```python
from build123d import *
from OCP.BRepFilletAPI import BRepFilletAPI_MakeChamfer

# Parameters (mm, degrees)
SKICA1_W                = 84
SKICA1_H                = 84
P_IDAT_VYSUNUT_M1_DEPTH = 2
SKICA1_3_W              = 80
SKICA1_3_H              = 80
SKICA1_3_W_2            = 37.6
SKICA1_3_H_2            = 76.8
SKICA1_3_H_3            = 37.6
P_IDAT_VYSUNUT_M2_DEPTH = 10.8
SKICA1_4_W              = 84
SKICA1_4_H              = 84
SKICA1_4_W_2            = 80
SKICA1_4_H_2            = 80
P_IDAT_VYSUNUT_M3_DEPTH = 4
ZKOSEN_2_SIZE           = 3.464101615
ZKOSEN_2_SIZE_2         = 2


with BuildPart() as part:
    # Skica1 → Přidat vysunutím1 (new body)
    with BuildSketch(Plane(origin=(0, 0, 0), x_dir=(1, 0, 0), z_dir=(0, 1, 0))):
        with Locations((-42, 42)):
            Rectangle(SKICA1_W, SKICA1_H)
    extrude(amount=P_IDAT_VYSUNUT_M1_DEPTH)

    # Skica1<3> → Přidat vysunutím2 (add)
    with BuildSketch(Plane(origin=(0, 0, 0), x_dir=(1, 0, 0), z_dir=(0, 1, 0))):
        with Locations((-42, 42)):
            Rectangle(SKICA1_3_W, SKICA1_3_H)
        with Locations((-22.4, 42)):
            Rectangle(SKICA1_3_W_2, SKICA1_3_H_2, mode=Mode.SUBTRACT)
        with Locations((-61.6, 61.6)):
            Rectangle(SKICA1_3_W_2, SKICA1_3_H_3, mode=Mode.SUBTRACT)
        with Locations((-61.6, 22.4)):
            Rectangle(SKICA1_3_W_2, SKICA1_3_H_3, mode=Mode.SUBTRACT)
    extrude(amount=P_IDAT_VYSUNUT_M2_DEPTH)

    # Skica1<4> → Přidat vysunutím3 (add)
    with BuildSketch(Plane(origin=(0, 0, 0), x_dir=(1, 0, 0), z_dir=(0, 1, 0))):
        with Locations((-42, 42)):
            Rectangle(SKICA1_4_W, SKICA1_4_H)
        with Locations((-42, 42)):
            Rectangle(SKICA1_4_W_2, SKICA1_4_H_2, mode=Mode.SUBTRACT)
    extrude(amount=P_IDAT_VYSUNUT_M3_DEPTH)

    # Zkosení2
    zkosen_2_edges_1 = [part.edges().sort_by_distance(p)[0] for p in [
        (-84, 4, -42),
    ]]
    zkosen_2_side_1 = [part.faces().sort_by_distance(p)[0] for p in [
        (-84, 3.96, -42),
    ]]
    zkosen_2_edges_2 = [part.edges().sort_by_distance(p)[0] for p in [
        (-42, 4, 0),
    ]]
    zkosen_2_side_2 = [part.faces().sort_by_distance(p)[0] for p in [
        (-42, 3.96, 0),
    ]]
    zkosen_2_edges_3 = [part.edges().sort_by_distance(p)[0] for p in [
        (0, 4, -42),
    ]]
    zkosen_2_side_3 = [part.faces().sort_by_distance(p)[0] for p in [
        (-0.04, 4, -42),
    ]]
    zkosen_2_edges_4 = [part.edges().sort_by_distance(p)[0] for p in [
        (-42, 4, -84),
    ]]
    zkosen_2_side_4 = [part.faces().sort_by_distance(p)[0] for p in [
        (-42, 3.96, -84),
    ]]
    zkosen_2 = BRepFilletAPI_MakeChamfer(part.part.solid().wrapped)
    for e in zkosen_2_edges_1:
        zkosen_2.Add(ZKOSEN_2_SIZE - 0.0001, ZKOSEN_2_SIZE_2 - 0.0001, e.wrapped, zkosen_2_side_1[0].wrapped)
    for e in zkosen_2_edges_2:
        zkosen_2.Add(ZKOSEN_2_SIZE - 0.0001, ZKOSEN_2_SIZE_2 - 0.0001, e.wrapped, zkosen_2_side_2[0].wrapped)
    for e in zkosen_2_edges_3:
        zkosen_2.Add(ZKOSEN_2_SIZE_2 - 0.0001, ZKOSEN_2_SIZE - 0.0001, e.wrapped, zkosen_2_side_3[0].wrapped)
    for e in zkosen_2_edges_4:
        zkosen_2.Add(ZKOSEN_2_SIZE - 0.0001, ZKOSEN_2_SIZE_2 - 0.0001, e.wrapped, zkosen_2_side_4[0].wrapped)
    add(Compound.cast(zkosen_2.Shape()), mode=Mode.REPLACE)  # a hair under: the kernel refuses the full size


solid = part.part
```
Here's how the part is built. I have some questions about the finished solid (model axes, mm). A direction names the side the tool comes from. Round coordinates to 2 decimals unless told otherwise and drop trailing zeros. Order: outer loops, then holes, each group sorted by start corner. A loop starts at its lowest first (then second) coordinate and runs counter-clockwise, first axis right, second up. Notation, with made-up numbers: M 24.25,40.5 L 49.25,40.5 A10 ccw 49.25,51.5 Z; hole C 75,2.5 d9. An arc over 180 degrees is marked long. One line per question, with ' | ' between items.
1) If we mould it in two halves opening along Z, with no side actions, what happens to faces 3 (the face through (-2, 7, -41)), 4 (the face through (-62, 6, -41.2)), 5 (the face through (-43, 7, -2))? For each: +Z half, -Z half, draft (parallel to the pull), parting line (faces both ways), or undercut.
Working result:
face 3: draft | face 4: undercut | face 5: +Z half
2) For pin 1 Ø6 at (x, y) = (-25.5, 4) entering from +Z; pin 2 Ø4.5 at (y, z) = (5, -36.5) entering from +X; pin 3 Ø5 at (x, y) = (-27, 5) entering from +Z, each with a flat end and sliding along its axis, tell me the tip position at first contact or that it passes through.
Working result:
pin 1: z = -0.27 | pin 2: x = -1.28 | pin 3: z = -1.13
3) I want a section at A-A, the plane y = 7.5. Write out the boundary of the cut face in (x, z).
Working result:
outline: M -82,-82 L -2,-82 L -2,-2 L -82,-2 Z; hole M -80.4,-80.4 L -42.8,-80.4 L -42.8,-42.8 L -80.4,-42.8 Z; hole M -80.4,-41.2 L -42.8,-41.2 L -42.8,-3.6 L -80.4,-3.6 Z; hole M -41.2,-80.4 L -3.6,-80.4 L -3.6,-3.6 L -41.2,-3.6 Z
4) For faces 1 (the face through (-42.588, 2.292, -82.986)), 2 (the face through (-23, 6, -80.4)), which set-ups out of +Z, -Z, +X, -X, +Y, -Y let a thin tool reach every point of the face, with its end or its side?
Working result:
face 1: -Z, +X, -X, +Y | face 2: +Y
5) I need wall thicknesses on line 1 along Z through (x, y) = (-53.5, 7); line 2 along Z through (x, y) = (-33.5, 6.25). Which ranges of each line are inside material? Lowest first, please.
Working result:
line 1: -82 to -80.4, -42.8 to -41.2, -3.6 to -2 | line 2: -82 to -80.4, -3.6 to -2
